Read the model definition and answer for the solid it produces. Units are mm, in the model's axes. Face numbers are marked on the shaded views. Give positions to 0.01 mm unless a question says otherwise; leave off trailing zeros. Loops run counter-clockwise (first coordinate to the right, second up) from the corner with the lowest first, then second, coordinate; pieces in that order, holes last.
(1) Find section B-B, the plane y = -165. Write down the section's boundary in (x, z).
(2) Determine the mould class of the marked faces 1 and 2 for opening direction Y: pulls with the +Y half, pulls with the -Y half, needs draft (parallel to the pull), parting line crosses it, or undercut.
(3) Straight lines are drawn through the part: probe 1 along X at (y, z) = (-210, 0.9); probe 2 along Y at (x, z) = (0, 6.35); probe 3 along Y at (x, z) = (160, 5.5). For each, find the intervals that lie inside material, in ascending order.
(4) Find section A-A, the plane x = -81. Write down the section's boundary in (y, z), then the cut area to 3 significant figures.
(5) Each of these flat-tipped pins is pushed along its axis until it touches: P1, Ø2, axis at y = 1.5, z = 6.5, coming from the +X side; P2, Ø1.7, axis at x = 0, y = -110, coming from the +Z side; P3, Ø4, axis at x = 124, y = -196.5, coming from the +Z side; P4, Ø0.5, axis at x = -1.5, z = 2.5, coming from the +Y side. Where does it stop, or does it pass through?
```python
from build123d import *

# Parameters (mm, degrees)
SKETCH_W        = 374
SKETCH_H        = 239
PAD_DEPTH       = 18
SKETCH001_W     = 344
SKETCH001_H     = 222
POCKET_DEPTH    = 15
SKETCH002_R     = 6
SKETCH002_R_2   = 7.5
PAD001_DEPTH    = 4
SKETCH003_R     = 1.45
HOLE_DEPTH      = 25
POCKET001_DEPTH = 4.5
SKETCH005_W     = 360
SKETCH005_H     = 230
POCKET002_DEPTH = 5
SKETCH006_W     = 7.9
SKETCH006_H     = 4.6
SKETCH006_W_2   = 9.8
SKETCH006_H_2   = 4.5
POCKET003_DEPTH = 2
SKETCH011_R     = 6
HOLE004_DEPTH   = 2
FILLET_R        = 5


with BuildPart() as part:
    # Sketch → Pad (new body)
    with BuildSketch(Plane.XY):
        with Locations((0, -117.5)):
            Rectangle(SKETCH_W, SKETCH_H)
    extrude(amount=PAD_DEPTH)

    # Sketch001 (on Face6 of Pad) → Pocket (cut)
    with BuildSketch(Plane.XY.offset(18)):
        with Locations((0, -111)):
            Rectangle(SKETCH001_W, SKETCH001_H)
    extrude(amount=-POCKET_DEPTH, mode=Mode.SUBTRACT)

    # Sketch002 (on Face11 of Pocket) → Pad001 (join)
    with BuildSketch(Plane.XY.offset(3)):
        with Locations((0, -110)):
            Circle(SKETCH002_R)
        with Locations((160, -10)):
            Circle(SKETCH002_R)
        with Locations((160, -210)):
            Circle(SKETCH002_R)
        with Locations((0, -210)):
            Circle(SKETCH002_R)
        with Locations((-160, -10)):
            Circle(SKETCH002_R_2)
        with Locations((-160, -210)):
            Circle(SKETCH002_R_2)
    extrude(amount=PAD001_DEPTH)

    # Sketch003 (on Face4 of Pad001) → Hole (cut)
    with BuildSketch(Plane(origin=(0, 0, 0), x_dir=(1, 0, 0), z_dir=(0, 0, -1))):
        with Locations((0, 110)):
            Circle(SKETCH003_R)
        with Locations((0, 210)):
            Circle(SKETCH003_R)
        with Locations((-160, 10)):
            Circle(SKETCH003_R)
        with Locations((-160, 210)):
            Circle(SKETCH003_R)
        with Locations((160, 10)):
            Circle(SKETCH003_R)
        with Locations((160, 210)):
            Circle(SKETCH003_R)
    extrude(amount=-HOLE_DEPTH, mode=Mode.SUBTRACT)

    # Sketch004 (on Face4 of Hole) → Pocket001 (cut)
    with BuildSketch(Plane(origin=(0, 0, 0), x_dir=(1, 0, 0), z_dir=(0, 0, -1))):
        Polygon((2.6, 111.501111), (0, 113.002221), (-2.6, 111.501111), (-2.6, 108.498889), (0, 106.997779), (2.6, 108.498889), align=None)
        Polygon((2.6, 208.498889), (2.6, 211.501111), (0, 213.002221), (-2.6, 211.501111), (-2.6, 208.498889), (0, 206.997779), align=None)
        Polygon((162.6, 208.498889), (162.6, 211.501111), (160, 213.002221), (157.4, 211.501111), (157.4, 208.498889), (160, 206.997779), align=None)
        Polygon((162.6, 8.498889), (162.6, 11.501111), (160, 13.002221), (157.4, 11.501111), (157.4, 8.498889), (160, 6.997779), align=None)
        Polygon((-157.4, 8.498889), (-157.4, 11.501111), (-160, 13.002221), (-162.6, 11.501111), (-162.6, 8.498889), (-160, 6.997779), align=None)
        Polygon((-157.4, 208.498889), (-157.4, 211.501111), (-160, 213.002221), (-162.6, 211.501111), (-162.6, 208.498889), (-160, 206.997779), align=None)
    extrude(amount=-POCKET001_DEPTH, mode=Mode.SUBTRACT)

    # Sketch005 (on Face5 of Pocket001) → Pocket002 (cut)
    with BuildSketch(Plane.XY.offset(18)):
        with Locations((0, -115)):
            Rectangle(SKETCH005_W, SKETCH005_H)
    extrude(amount=-POCKET002_DEPTH, mode=Mode.SUBTRACT)

    # Sketch006 (on Pad) → Pocket003 (cut)
    with BuildSketch(Plane.XZ):
        with BuildLine():
            ThreePointArc((-2.6, 8.9), (-6, 5.5), (-2.6, 2.1))
            Line((-2.6, 2.1), (2.6, 2.1))
            ThreePointArc((2.6, 2.1), (6, 5.5), (2.6, 8.9))
            Line((2.6, 8.9), (-2.6, 8.9))
        make_face()
        with Locations((56.5, 5.5)):
            Rectangle(SKETCH006_W, SKETCH006_H)
        with Locations((42, 5.5)):
            Rectangle(SKETCH006_W_2, SKETCH006_H_2)
    extrude(amount=-POCKET003_DEPTH, mode=Mode.SUBTRACT)

    # Sketch011 (on Face4 of Pad001) → Hole004 (cut)
    with BuildSketch(Plane(origin=(0, 0, 0), x_dir=(1, 0, 0), z_dir=(0, 0, -1))):
        with Locations((0, 110)):
            Circle(SKETCH011_R)
        with Locations((0, 210)):
            Circle(SKETCH011_R)
        with Locations((-160, 10)):
            Circle(SKETCH011_R)
        with Locations((-160, 210)):
            Circle(SKETCH011_R)
        with Locations((160, 10)):
            Circle(SKETCH011_R)
        with Locations((160, 210)):
            Circle(SKETCH011_R)
    extrude(amount=-HOLE004_DEPTH, mode=Mode.SUBTRACT)

    # Fillet
    fillet_edges = [part.edges().sort_by_distance(p)[0] for p in [
        (-187, 2, 9),
        (-187, -237, 9),
        (187, 2, 9),
        (187, -237, 9),
    ]]
    fillet(fillet_edges, radius=FILLET_R)


solid = part.part
```
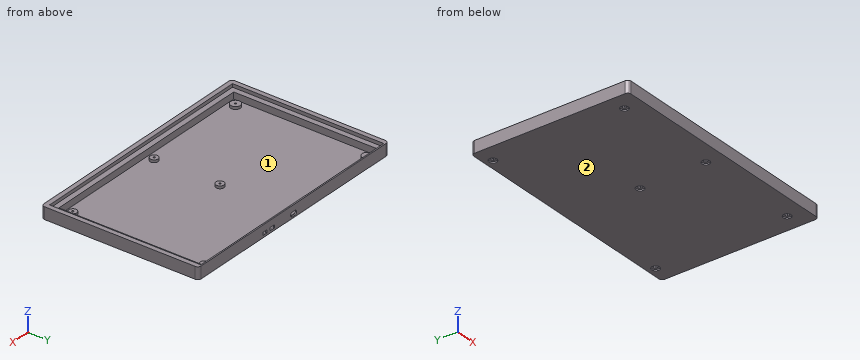
Entries:
1. outline: (-187, 0) - (187, 0) - (187, 18) - (180, 18) - (180, 13) - (172, 13) - (172, 3) - (-172, 3) - (-172, 13) - (-180, 13) - (-180, 18) - (-187, 18) - close
2. face 1: undercut
2. face 2: needs draft
3. probe 1: x = -187 to -166, -154 to -6, 6 to 154, 166 to 187
3. probe 2: y = -237 to -222, -216 to -211.45, -208.55 to -204, -116 to -111.45, -108.55 to -104
3. probe 3: y = -237 to -222, -216 to -211.45, -208.55 to -204, -16 to -11.45, -8.55 to -4, 0 to 2
4. outline: (-237, 0) - (2, 0) - (2, 18) - (0, 18) - (0, 3) - (-222, 3) - (-222, 13) - (-230, 13) - (-230, 18) - (-237, 18) - close
4. area: 932 mm2
5. P1: stops at x = 185.57
5. P2: passes through
5. P3: stops at z = 3
5. P4: stops at y = 0
